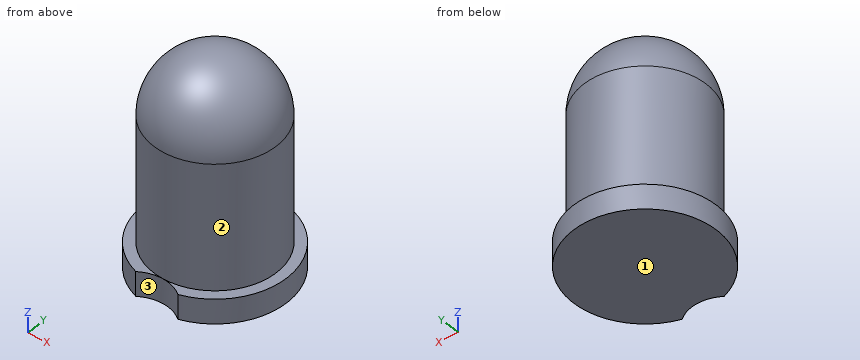
from build123d import *

# Parameters (mm, degrees)
SKETCH1_R                = 2.5
SKETCH1_R_2              = 2
BOSS_EXTRUDE1_DEPTH      = 5.1
SKETCH3_R                = 2.925
BOSS_EXTRUDE2_DEPTH      = 1
SKETCH4_R                = 2
CUT_EXTRUDE2_DEPTH       = 5.1
BOSS_EXTRUDE3_DEPTH      = 0.3
BOSS_EXTRUDE3_DEPTH_BACK = 0.3
SKETCH9_R                = 1.5
CUT_EXTRUDE3_DEPTH       = 3


with BuildPart() as part:
    # Sketch1 → Boss-Extrude1 (new body)
    with BuildSketch(Plane.XY):
        Circle(SKETCH1_R)
        Circle(SKETCH1_R_2, mode=Mode.SUBTRACT)
    extrude(amount=BOSS_EXTRUDE1_DEPTH)

    # Sketch2 → Revolve1 (revolve)
    with BuildSketch(Plane.XY.offset(5.1)):
        with BuildLine():
            Line((-2.5, 0), (-2, 0))
            ThreePointArc((-2, 0), (0, -2), (2, 0))
            Line((2, 0), (2.5, 0))
            ThreePointArc((2.5, 0), (0, -2.5), (-2.5, 0))
        make_face()
    revolve(axis=Axis((-3.079262147, 0, 5.1), (1, 0, 0)))

    # Sketch3 → Boss-Extrude2 (add)
    with BuildSketch(Plane(origin=(0, 0, 0), x_dir=(-1, 0, 0), z_dir=(0, 0, -1))):
        Circle(SKETCH3_R)
    extrude(amount=BOSS_EXTRUDE2_DEPTH)

    # Sketch4 → Cut-Extrude2 (cut)
    with BuildSketch(Plane.XY):
        Circle(SKETCH4_R)
    extrude(amount=CUT_EXTRUDE2_DEPTH, mode=Mode.SUBTRACT)

    # Sketch6 → Boss-Extrude3 (add, two sides: drawn at the far end of the back side and taken through both)
    with BuildSketch(Plane(origin=(0, 0, 0), x_dir=(0, 0, -1), z_dir=(1, 0, 0)).offset(-BOSS_EXTRUDE3_DEPTH_BACK)):
        Polygon((0, 1.206894491), (-3.556166294, 1.206894491), (-3.556166294, -0.084621026), (-2.37503672, 0.643926189), (-2.37503672, 0.897813854), (0, 0.897813854), align=None)
        Polygon((-3.556166294, -0.28331572), (-3.330966178, -0.28331572), (-3.330966178, -0.18084552), (-2.37503672, 0.4341929), (-2.37503672, -0.28331572), (0, -0.28331572), (0, -0.780052457), (-3.556166294, -0.780052457), align=None)
    extrude(amount=BOSS_EXTRUDE3_DEPTH + BOSS_EXTRUDE3_DEPTH_BACK)

    # Sketch9 → Cut-Extrude3 (cut)
    with BuildSketch(Plane.XY):
        with Locations((0, -4)):
            Circle(SKETCH9_R)
    extrude(amount=-CUT_EXTRUDE3_DEPTH, mode=Mode.SUBTRACT)


solid = part.part
CAD build for the part. Positions are in the model's coordinates, mm. Face numbers are marked on the shaded views. Round coordinates to 2 decimals unless told otherwise and drop trailing zeros. Write each loop counter-clockwise with the first axis right and the second up, starting at its lowest first coordinate (ties: lowest second). Pieces come first, ordered by that corner, then holes. Notation, with made-up numbers: M 4,16 L 52,16 A27 ccw 52,46 Z; hole C 60,60 d8. An arc over 180 degrees is marked long. Use a Markdown table: item, result. Add a question column.
1. Slice it at B-B on x = 1.4. Give the cut face in (y, z), then the cut area to 3 significant figures.
2. Slice it at C-C on y = -1.65. Give the cut face in (x, z), then the cut area to 3 significant figures.
3. Drill centre lines: probe 1 along X at (y, z) = (0, 2.5); probe 2 along Y at (x, z) = (0, 0.8); probe 3 along Y at (x, z) = (0, 4.1). Where is each one in solid material? Low to high.
4. Flat gauge pins, fed straight in: P1, Ø0.7, axis at x = 0, z = 0.5, coming from the +Y side; P2, Ø1, axis at y = 0.5, z = 1.5, coming from the -X side; P3, Ø0.5, axis at x = 0, y = 0.5, coming from the +Z side. Where does each tip first touch, or does it go through?
5. Pull direction X, two halves, no side cores. Call the marked faces 1, 2 and 3: released by +X, released by -X, zero draft, split by the parting line, or undercut.
6. Slice it at A-A on z = 3. Give the cut face in (x, y).
7. Slice it at D-D on x = 2.3. Give the cut face in (y, z).
Reply:
| question | item | result |
|---|---|---|
| 1 | outline | M -2.57,-1 L 2.57,-1 L 2.57,0 L 2.07,0 L 2.07,5.1 A2.07 ccw -2.07,5.1 L -2.07,0 L -2.57,0 Z; hole M -1.43,0 L 1.43,0 L 1.43,5.1 A1.43 ccw -1.43,5.1 Z |
| 1 | area | 15.2 mm^2 |
| 2 | outline | M -2.42,-1 L 2.42,-1 L 2.42,0 L 1.88,0 L 1.88,5.1 A1.88 ccw -1.88,5.1 L -1.88,0 L -2.42,0 Z; hole M -1.13,0 L 1.13,0 L 1.13,5.1 A1.13 ccw -1.13,5.1 Z |
| 2 | area | 16.0 mm^2 |
| 3 | probe 1 | x = -2.5 to -2, -0.3 to 0.3, 2 to 2.5 |
| 3 | probe 2 | y = -2.5 to -2, -0.78 to -0.28, 0.9 to 1.21, 2 to 2.5 |
| 3 | probe 3 | y = -2.5 to -2, 2 to 2.5 |
| 4 | P1 | stops at y = 2.5 |
| 4 | P2 | stops at x = -2.5 |
| 4 | P3 | stops at z = 7.59 |
| 5 | face 1 | zero draft |
| 5 | face 2 | split by the parting line |
| 5 | face 3 | undercut |
| 6 | outline | C 0,0 d5; M -0.3,-0.78 L 0.3,-0.78 L 0.3,0.03 L -0.3,0.03 Z; M -0.3,0.26 L 0.3,0.26 L 0.3,1.21 L -0.3,1.21 Z; hole C 0,0 d4 |
| 7 | outline | M -1.81,-1 L 1.81,-1 L 1.81,0 L 0.98,0 L 0.98,5.1 A0.98 ccw -0.98,5.1 L -0.98,0 L -1.81,0 Z |
